Autodesk Inventor part; units mm, degrees
ref_plane "YZ Plane" through (0, 0, 0) normal (1, 0, 0) x (0, 1, 0)
ref_plane "XZ Plane" through (0, 0, 0) normal (0, 1, 0) x (-1, 0, 0)
ref_plane "XY Plane" through (0, 0, 0) normal (0, 0, 1) x (1, 0, 0)
sketch "Boceto1" plane through (0, 0, 0) normal (0, 0, 1) x (1, 0, 0)
  circle A0 centre (0, 0) radius 10
  dimension "d0" = 20
extrude "Extrusión1" add sketch "Boceto1" along normal blind 4
sketch "Boceto2" plane through (0, 0, 4) normal (0, 0, 1) x (1, 0, 0)
  circle A0 centre (0, 0) radius 6.5
  dimension "d3" = 13
extrude "Extrusión2" add sketch "Boceto2" along normal blind 50
sketch "Boceto3" plane through (0, 0, 0) normal (0, 1, 0) x (-1, 0, 0)
  line L0 (6.5, 50) -> (5.5, 50)
  line L1 (5.5, 50) -> (5.5, 8)
  line L2 (5.5, 8) -> (6.5, 8)
  line L3 (0, 30.7495) -> (0, -2.427)
  line L4 (10, 4) -> (-10, 4)
  line L5 (6.5, 4) -> (6.5, 54)
  point P0 (0, 0)
  dimension "d6" = 1
  dimension "d7" = 4
  dimension "d8" = 4
revolve "Revolución1" cut sketch "Boceto3" angle 360 about axis through (0, 0, 30.7495) along (0, 0, -1)
sketch "Boceto4" plane through (0, 0, 54) normal (0, 0, 1) x (1, 0, 0)
  circle A0 centre (0, 0) radius 3
  dimension "d10" = 6
extrude "Extrusión3" cut sketch "Boceto4" against normal blind 10
properties part number "steering_stand_off_bush" material "Hierro, gris"
The listing builds one solid part. Answer for the finished solid, in the listing's coordinates (mm). A direction names the side the tool comes from. Give positions to 0.01 mm unless a question says otherwise; leave off trailing zeros. Write each loop counter-clockwise with the first axis right and the second up, starting at its lowest first coordinate (ties: lowest second). Pieces come first, ordered by that corner, then holes.
Item 1: Section A-A, the plane x = -6 is taken. Write down the section's boundary in (y, z), plus the area to 3 significant figures.
Item 2: Determine the mould class of faces 1 (the flat face through (0, 0, 44)), 2 (the flat face through (3, -1, 54)), 3 (the cylindrical face through (1.19, -5.37, 28.71)) for opening direction Y: released by +Y, released by -Y, zero draft, split by the parting line, or undercut.
Item 3: Section B-B, the plane y = 0 is taken. Write down the section's boundary in (x, z).
Item 4: Find the intervals of material crossed by line 1 along Y through (x, z) = (0, 50.5); line 2 along Z through (x, y) = (-6.25, -3); line 3 along Y through (x, z) = (0, 47.5), in increasing order.
Item 5: Section C-C, the plane z = 46.5 is taken. Write down the section's boundary in (x, y).
Item 6: Flat-ended cylindrical pins translate along their axes: P1, Ø1.5, axis at y = -3.5, z = 17.5, coming from the -X side; P2, Ø1, axis at y = -1.5, z = 12.5, coming from the +X side; P3, Ø1.5, axis at x = 2.5, z = 39, coming from the +Y side. Find the tip coordinate at first contact, or state that the pin passes through.
Item 7: Which of the six approach directions +Z, -Z, +X, -X, +Y, -Y give full straight-line access (tool end or side, diameter ignored) to faces 4 (the flat face through (5, 3, 50)), 5 (the flat face through (7, 0, 4)), 6 (the flat face through (0, 0, 0))?
Completed:
1. outline: (-8, 0) - (8, 0) - (8, 4) - (2.5, 4) - (2.5, 8) - (-2.5, 8) - (-2.5, 4) - (-8, 4) - close; (-2.5, 50) - (2.5, 50) - (2.5, 54) - (-2.5, 54) - close
1. area: 104 mm2
2. face 1: undercut
2. face 2: zero draft
2. face 3: split by the parting line
3. outline: (-10, 0) - (10, 0) - (10, 4) - (6.5, 4) - (6.5, 8) - (5.5, 8) - (5.5, 50) - (6.5, 50) - (6.5, 54) - (3, 54) - (3, 44) - (-3, 44) - (-3, 54) - (-6.5, 54) - (-6.5, 50) - (-5.5, 50) - (-5.5, 8) - (-6.5, 8) - (-6.5, 4) - (-10, 4) - close
4. line 1: y = -6.5 to -3, 3 to 6.5
4. line 2: z = 0 to 4
4. line 3: y = -5.5 to -3, 3 to 5.5
5. outline: circle Ø11 at (0, 0); hole circle Ø6 at (0, 0)
6. P1: stops at x = -4.76
6. P2: stops at x = 5.41
6. P3: stops at y = 5.21
7. face 4: none
7. face 5: +Z
7. face 6: -Z, +X, -X, +Y, -Y
